Check sheet for the modelled part. Datum: model origin and axes. Units: mm. Face numbers are marked on the shaded views. A direction names the side the tool comes from. Round coordinates to 2 decimals unless told otherwise and drop trailing zeros. Loops run counter-clockwise (first coordinate to the right, second up) from the corner with the lowest first, then second, coordinate; pieces in that order, holes last. Notation, with made-up numbers: (-22.5, 26.25) - (25.5, 26.25) arc R25 ccw to (25.5, 44.25) - close; hole circle Ø7 at (-20, -35). An arc over 180 degrees is marked (long way). Put each result on its own line as item: value.
```python
from build123d import *

# Parameters (mm, degrees)
SKETCH_R        = 5
SKETCH_R_2      = 3.2
PAD_DEPTH       = 15
SKETCH002_R     = 6.1
POCKET001_DEPTH = 4
SKETCH003_R     = 11.1
POCKET_DEPTH    = 7.4


with BuildPart() as part:
    # Sketch → Pad (new body)
    with BuildSketch(Plane.XY):
        Polygon((20, 30), (20, 50.15), (62.3, 50.15), (62.3, 30), (82.3, 30), (82.3, 0), (0, 0), (0, 30), align=None)
        with Locations((41.15, 29)):
            Circle(SKETCH_R, mode=Mode.SUBTRACT)
        with Locations((11.15, 10)):
            Circle(SKETCH_R_2, mode=Mode.SUBTRACT)
        with Locations((31.15, 10)):
            Circle(SKETCH_R_2, mode=Mode.SUBTRACT)
        with Locations((51.15, 10)):
            Circle(SKETCH_R_2, mode=Mode.SUBTRACT)
        with Locations((71.15, 10)):
            Circle(SKETCH_R_2, mode=Mode.SUBTRACT)
    extrude(amount=PAD_DEPTH)

    # Sketch002 → Pocket001 (cut)
    with BuildSketch(Plane(origin=(0, 0, 0), x_dir=(1, 0, 0), z_dir=(0, 0, -1))):
        with Locations((11.15, -10)):
            Circle(SKETCH002_R)
        with Locations((31.15, -10)):
            Circle(SKETCH002_R)
        with Locations((51.15, -10)):
            Circle(SKETCH002_R)
        with Locations((71.15, -10)):
            Circle(SKETCH002_R)
    extrude(amount=-POCKET001_DEPTH, mode=Mode.SUBTRACT)

    # Sketch003 (on Face5 of Pocket001) → Pocket (cut)
    with BuildSketch(Plane.XY.offset(15)):
        with Locations((41.15, 29)):
            Circle(SKETCH003_R)
    extrude(amount=-POCKET_DEPTH, mode=Mode.SUBTRACT)


solid = part.part
```
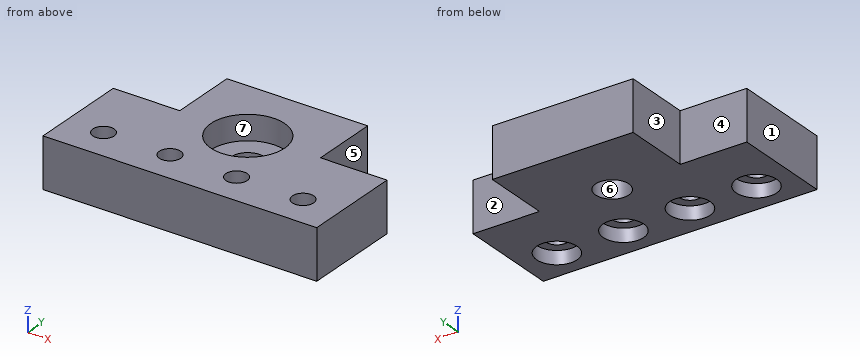
Item 1: Go/stop test with flat-tipped pins: pin 1 (7.5 mm diameter, centred on y = 41, z = 9.5, fed in from +X); pin 2 (6 mm diameter, centred on x = 8.5, y = 10, fed in from -Z); pin 3 (5 mm diameter, centred on x = 68.5, z = 2.5, fed in from +Y). Record where each tip stops, or that it passes through.
Filled sheet:
pin 1: x = 62.3
pin 2: z = 4
pin 3: y = 30
Item 2: Tool access check on the marked faces 1, 2 and 3. Record the directions out of +Z, -Z, +X, -X, +Y, -Y that give a thin tool (end or side, any length) a straight path to the whole face; none if there is none.
Filled sheet:
face 1: +Z, -Z, -X, +Y, -Y
face 2: +Z, -Z, +X, +Y
face 3: +Z, -Z, -X, +Y
Item 3: Section check B-B on x = 41.15. Enter the section's corners in (y, z).
Filled sheet:
outline: (0, 0) - (24, 0) - (24, 7.6) - (17.9, 7.6) - (17.9, 15) - (0, 15) - close; (34, 0) - (50.15, 0) - (50.15, 15) - (40.1, 15) - (40.1, 7.6) - (34, 7.6) - close
Item 4: Release check for a two-part mould opening along X. For the marked faces 4, 5, 6 and 7 record: +X half, -X half, draft (parallel to the pull), parting line (faces both ways), or undercut.
Filled sheet:
face 4: draft
face 5: +X half
face 6: undercut
face 7: undercut
Item 5: Section check D-D on x = 51.15. Enter the section's corners in (y, z), then the cut area to 3 significant figures.
Filled sheet:
outline: (0, 0) - (3.9, 0) - (3.9, 4) - (6.8, 4) - (6.8, 15) - (0, 15) - close; (13.2, 4) - (16.1, 4) - (16.1, 0) - (50.15, 0) - (50.15, 15) - (33.82, 15) - (33.82, 7.6) - (24.18, 7.6) - (24.18, 15) - (13.2, 15) - close
area: 562 mm²
Item 6: Thickness scan on line 1 (X direction, y = 10, z = 2.3); line 2 (X direction, y = 10, z = 11.5); line 3 (X direction, y = 29, z = 6.25). Record the ranges inside material, lowest first. Write a range as from..to.
Filled sheet:
line 1: 0..5.05, 17.25..25.05, 37.25..45.05, 57.25..65.05, 77.25..82.3
line 2: 0..7.95, 14.35..27.95, 34.35..47.95, 54.35..67.95, 74.35..82.3
line 3: 0..36.15, 46.15..82.3
Item 7: Section check C-C on y = 10. Count the separate pieces of the cut face and the enclosed holes in it, then the cut area to 3 significant figures.
Filled sheet:
separate pieces: 5
enclosed holes: 0
area: 758 mm²
Item 8: Section check A-A on y = 29. Enter the section's corners in (x, z).
Filled sheet:
outline: (0, 0) - (36.15, 0) - (36.15, 7.6) - (30.05, 7.6) - (30.05, 15) - (0, 15) - close; (46.15, 0) - (82.3, 0) - (82.3, 15) - (52.25, 15) - (52.25, 7.6) - (46.15, 7.6) - close
